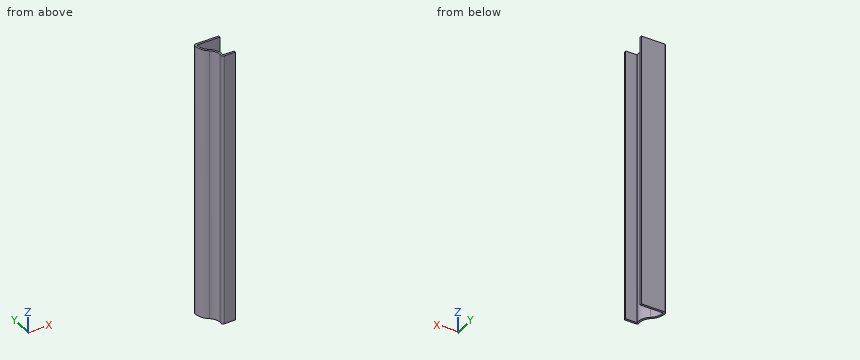
```python
from build123d import *

# Parameters (mm, degrees)
EXTRUDE_THIN1_DEPTH = 142.875
FILLET1_R           = 1.016


with BuildPart() as part:
    # Sketch1 → Extrude-Thin1 (new body)
    with BuildSketch(Plane.XY):
        with BuildLine():
            Line((0, 0), (-6.746875, 0))
            Line((-6.746875, 0), (-6.746875, 1.919148688))
            ThreePointArc((-6.746875, 1.919148688), (-7.41996004, 4.62577026), (-9.28241202, 6.70185225))
            ThreePointArc((-9.28241202, 6.70185225), (-12.064724111, 10.011020322), (-12.7, 14.2875))
            Line((-12.7, 14.2875), (0, 14.2875))
            Line((0, 14.2875), (0, 13.2715))
            Line((0, 13.2715), (-11.749292543, 13.2715))
            ThreePointArc((-11.749292543, 13.2715), (-10.943069803, 10.029502732), (-8.712220727, 7.542767162))
            ThreePointArc((-8.712220727, 7.542767162), (-6.522304662, 5.101659767), (-5.730875, 1.919148688))
            Line((-5.730875, 1.919148688), (-5.730875, 1.016))
            Line((-5.730875, 1.016), (0, 1.016))
            Line((0, 1.016), (0, 0))
        make_face()
    extrude(amount=-EXTRUDE_THIN1_DEPTH)

    # Fillet1
    fillet1_edges = [part.edges().sort_by_distance(p)[0] for p in [
        (-6.746875, 0, -71.4375),
        (-12.7, 14.2875, -71.4375),
    ]]
    fillet(fillet1_edges, radius=FILLET1_R)


solid = part.part
```
Work out the finished part from the listing and answer in its coordinate system (mm). Coordinates: 2 decimals unless noted, no trailing zeros. Write each loop counter-clockwise with the first axis right and the second up, starting at its lowest first coordinate (ties: lowest second). Pieces come first, ordered by that corner, then holes.
Q1. A cutting plane is placed at C-C, the plane y = 4. Give the vertices of the cut face in (x, z) (3 decimals), then the cut area to 3 significant figures.
Q2. A cutting plane is placed at A-A, the plane x = -3.25. Give the vertices of the cut face in (y, z) (1 decimal), then the cut area to 3 significant figures.
Q3. Each of these flat-tipped pins is pushed along its axis until it touches: pin 1 Ø1 at (x, z) = (-10, -120.5) entering from -Y; pin 2 Ø1 at (y, z) = (1.5, -45.5) entering from -X; pin 3 Ø5 at (y, z) = (6, -116.5) entering from -X. Where does it stop, or does it pass through?
Q4. A cutting plane is placed at B-B, the plane z = -32.5. Give the vertices of the cut face in (x, y) (1 decimal).
Q5. Find the intervals of material crossed by line 1 (Y direction, x = -3.5, z = -72.5); line 2 (Y direction, x = -10.75, z = -16); line 3 (X direction, y = 13.5, z = -40.5), in increasing order.
Findings below:
1. outline: (-7.135, -142.875) - (-6.057, -142.875) - (-6.057, 0) - (-7.135, 0) - close
1. area: 154 mm2
2. outline: (0, -142.9) - (1, -142.9) - (1, 0) - (0, 0) - close; (13.3, -142.9) - (14.3, -142.9) - (14.3, 0) - (13.3, 0) - close
2. area: 290 mm2
3. pin 1: stops at y = 6.85
3. pin 2: stops at x = -6.75
3. pin 3: stops at x = -11.17
4. outline: (-12.8, 13.3) arc R7.9 ccw to (-9.3, 6.7) arc R5.8 cw to (-6.7, 1.9) - (-6.7, 1) arc R1 ccw to (-5.7, 0) - (0, 0) - (0, 1) - (-5.7, 1) - (-5.7, 1.9) arc R6.8 ccw to (-8.7, 7.5) arc R6.9 cw to (-11.7, 13.3) - (0, 13.3) - (0, 14.3) - (-11.7, 14.3) arc R1 ccw to start
5. line 1: y = 0 to 1.02, 13.27 to 14.29
5. line 2: y = 7.99 to 9.69, 13.27 to 14.29
5. line 3: x = -12.74 to 0
